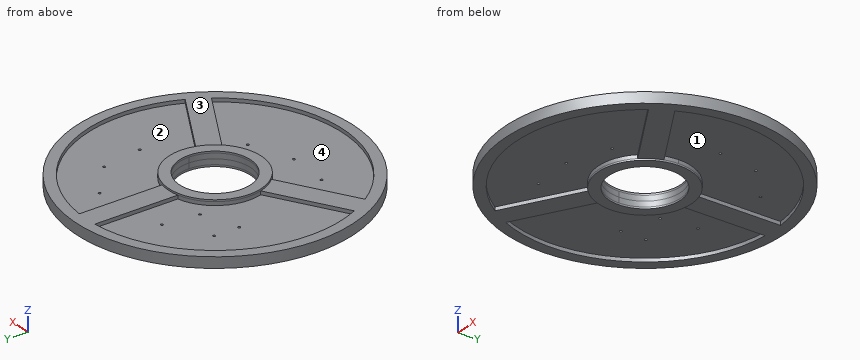
Solid Edge part; units mm, degrees
sketch "Sketch1" plane through (0, 0, 0) normal (0, 0, -1) x (-1, 0, 0)
  circle A0 centre (0, 0) radius 5
  arc A1 (4.7272, -4.4613) -> (-4.7325, -4.4557) centre (0, 0) cw
  line L0 (-14.7885, -10.2616) -> (-4.7325, -4.4557)
  arc A2 (14.7842, -10.2677) -> (-14.7885, -10.2616) centre (0, 0) cw
  line L1 (14.7842, -10.2677) -> (4.7272, -4.4613)
  line L2 (16.2842, -7.6697) -> (6.2272, -1.8632)
  arc A3 (1.5, 17.9374) -> (16.2842, -7.6697) centre (0, 0) cw
  line L3 (1.5, 17.9374) -> (1.5, 6.3246)
  arc A4 (1.5, 6.3246) -> (6.2272, -1.8632) centre (0, 0) cw
  arc A5 (-6.2272, -1.8632) -> (-1.5, 6.3246) centre (0, 0) cw
  line L4 (-1.5, 17.9374) -> (-1.5, 6.3246)
  line L5 (-16.2842, -7.6697) -> (-6.2272, -1.8632)
  arc A6 (-16.2842, -7.6697) -> (-1.5, 17.9374) centre (0, 0) cw
  circle A7 centre (0, 0) radius 19.5
extrude "Protrusion1" add sketch "Sketch1" along normal mid plane 1.5
sketch "Sketch2" plane through (0, 0, 0) normal (0, 0, 1) x (1, 0, 0)
  circle A0 centre (0, 0) radius 5
  circle A1 centre (0, 0) radius 6.5
extrude "Kihúzás_2" add sketch "Sketch2" along normal mid plane 2
sketch "Sketch3" plane through (0, 0, 0) normal (0, 0, 1) x (1, 0, 0)
  arc A0 (-16.2842, -7.6697) -> (-1.5, 17.9374) centre (0, 0) cw
  line L0 (-1.5, 17.9374) -> (-1.5, 6.3246)
  arc A1 (-1.5, 6.3246) -> (-6.2272, -1.8632) centre (0, 0) ccw
  line L1 (-6.2272, -1.8632) -> (-16.2842, -7.6697)
  line L2 (1.5, 6.3246) -> (1.5, 17.9374)
  arc A2 (1.5, 17.9374) -> (16.2842, -7.6697) centre (0, 0) cw
  line L3 (16.2842, -7.6697) -> (6.2272, -1.8632)
  arc A3 (6.2272, -1.8632) -> (1.5, 6.3246) centre (0, 0) ccw
  line L4 (4.7325, -4.4557) -> (14.7885, -10.2616)
  arc A4 (14.7885, -10.2616) -> (-14.7842, -10.2677) centre (0, 0) cw
  line L5 (-14.7842, -10.2677) -> (-4.7272, -4.4613)
  arc A5 (-4.7272, -4.4613) -> (4.7325, -4.4557) centre (0, 0) ccw
extrude "Kihúzás_3" add sketch "Sketch3" along normal mid plane 0.5
hole "Furat_1" at (-10.961, 8.1069, 0.25) direction (0, 0, -1) diameter 0.35 end up to next
hole "Hole1" at (-10.9869, 4.6272, 0.25) direction (0, 0, -1) diameter 0.35 end up to next
hole "Hole2" at (-5.3514, 11.3456, 0.25) direction (0, 0, -1) diameter 0.35 end up to next
hole "Hole3" at (-5.9322, 6.4456, 0.25) direction (0, 0, -1) diameter 0.35 end up to next
hole "Hole4" at (4.8333, 12.6611, 0.25) direction (0, 0, -1) diameter 0.35 end up to next
hole "Hole5" at (9.5361, 8.6117, 0.25) direction (0, 0, -1) diameter 0.35 end up to next
hole "Hole6" at (10.4296, 2.968, 0.25) direction (0, 0, -1) diameter 0.35 end up to next
hole "Hole7" at (-1.6476, -9.8344, 0.25) direction (0, 0, -1) diameter 0.35 end up to next
hole "Hole8" at (-7.4503, -9.4999, 0.25) direction (0, 0, -1) diameter 0.35 end up to next
hole "Hole9" at (4.1734, -7.6286, 0.25) direction (0, 0, -1) diameter 0.35 end up to next
properties material "Plastic ABS (medium strong)"
Here's how the part is built. I have some questions about the finished solid (model axes, mm). Face numbers are marked on the shaded views. A direction names the side the tool comes from. Give positions to 0.01 mm unless a question says otherwise; leave off trailing zeros. Order: outer loops, then holes, each group sorted by start corner. A loop starts at its lowest first (then second) coordinate and runs counter-clockwise, first axis right, second up. Notation, with made-up numbers: M -25,69.5 L -4,69.5 A14 ccw -4,84.5 Z; hole C 42.5,28 d7. An arc over 180 degrees is marked long. Use a Markdown table: item, result. Add a question column.
1. On a 3-axis mill with a long thin cutter (end or side, diameter ignored), from which of +Z, -Z, +X, -X, +Y, -Y can I reach the whole of each face in a straight line? I mean the marked faces 1 and 2. Say none if no direction works.
2. Suppose I cut it at A-A (x = 0). List the corners of the cut face in (y, z) for me, and give its area (3 significant figures).
3. Suppose I cut it at C-C (x = -17). List the corners of the cut face in (y, z) for me, and give its area (3 significant figures).
4. Suppose I cut it at D-D (y = -14.5). List the corners of the cut face in (x, z) for me, and give its area (3 significant figures).
5. I need wall thicknesses on probe 1 along X at (y, z) = (13.5, -0.4); probe 2 along X at (y, z) = (15.5, 0.55); probe 3 along X at (y, z) = (-2.5, 0.35). Which ranges of each line are inside material? Lowest first, please. Write a range as from..to.
6. Suppose I cut it at B-B (y = -1). List the corners of the cut face in (x, z) for me.
7. If we mould it in two halves opening along X, with no side actions, what happens to the marked faces 3 and 4? For each: +X half, -X half, draft (parallel to the pull), parting line (faces both ways), or undercut.
8. For pin 1 Ø1 at (y, z) = (8.5, 0) entering from +X; pin 2 Ø5 at (x, y) = (10, 1.5) entering from +Z; pin 3 Ø15 at (x, y) = (5, -9.5) entering from -Z; pin 4 Ø6 at (x, y) = (13, 11.5) entering from -Z, each with a flat end and sliding along its axis, tell me the tip position at first contact or that it passes through.
Results list:
| question | item | result |
|---|---|---|
| 1 | face 1 | -Z |
| 1 | face 2 | +Z |
| 2 | outline | M -19.5,-0.75 L -18,-0.75 L -18,-0.25 L -6.5,-0.25 L -6.5,-1 L -5,-1 L -5,1 L -6.5,1 L -6.5,0.25 L -18,0.25 L -18,0.75 L -19.5,0.75 Z; M 5,-1 L 6.5,-1 L 6.5,-0.75 L 19.5,-0.75 L 19.5,0.75 L 6.5,0.75 L 6.5,1 L 5,1 Z |
| 2 | area | 33.5 mm² |
| 3 | outline | M -9.55,-0.75 L -5.92,-0.75 L -5.92,-0.25 L 5.92,-0.25 L 5.92,-0.75 L 9.55,-0.75 L 9.55,0.75 L 5.92,0.75 L 5.92,0.25 L -5.92,0.25 L -5.92,0.75 L -9.55,0.75 Z |
| 3 | area | 16.8 mm² |
| 4 | outline | M -13.04,-0.75 L -10.67,-0.75 L -10.67,-0.25 L 10.67,-0.25 L 10.67,-0.75 L 13.04,-0.75 L 13.04,0.75 L 10.67,0.75 L 10.67,0.25 L -10.67,0.25 L -10.67,0.75 L -13.04,0.75 Z |
| 4 | area | 17.8 mm² |
| 5 | probe 1 | x = -14.07..-11.91, -1.5..1.5, 11.91..14.07 |
| 5 | probe 2 | x = -11.83..-9.15, -1.5..1.5, 9.15..11.83 |
| 5 | probe 3 | x = -19.34..-17.83, -7.33..-4.33, 4.33..7.33, 17.83..19.34 |
| 6 | outline | M -19.47,-0.75 L -17.97,-0.75 L -17.97,-0.25 L -6.42,-0.25 L -6.42,-1 L -4.9,-1 L -4.9,1 L -6.42,1 L -6.42,0.25 L -17.97,0.25 L -17.97,0.75 L -19.47,0.75 Z; M 4.9,-1 L 6.42,-1 L 6.42,-0.25 L 17.97,-0.25 L 17.97,-0.75 L 19.47,-0.75 L 19.47,0.75 L 17.97,0.75 L 17.97,0.25 L 6.42,0.25 L 6.42,1 L 4.9,1 Z |
| 7 | face 3 | draft |
| 7 | face 4 | undercut |
| 8 | pin 1 | stops at x = 17.78 |
| 8 | pin 2 | stops at z = 0.25 |
| 8 | pin 3 | stops at z = -1 |
| 8 | pin 4 | stops at z = -0.75 |
